The figure shows three views and two pictorial views of one solid part (mm, origin at its lowest corner). Answer the questions. Give positions to 0.01 mm unless a question says otherwise; leave off trailing zeros. Loops run counter-clockwise (first coordinate to the right, second up) from the corner with the lowest first, then second, coordinate; pieces in that order, holes last. Notation, with made-up numbers: M 56,-19 L 70,-19 A10 cw 70,-2 Z; hole C 73,12 d1. An arc over 180 degrees is marked long. Write item = value, one per line. Start each with the question number.
1. Section A-A on y = 1.05 is taken. Determine the outline of the cut face in (x, z).
2. Section B-B on z = 2 is taken. Determine the outline of the cut face in (x, y).
3. Consider L1, parallel to Z at x = 16, y = 0.7; L2, parallel to X at y = 0.2, z = 2.5; L3, parallel to Z at x = 38, y = 0.75. Determine where each line is inside the solid, lowest interval first. Write a range as [from, to].
4. Section D-D on x = 29 is taken. Determine the outline of the cut face in (y, z).
5. Section C-C on z = 5.25 is taken. Determine the outline of the cut face in (x, y).
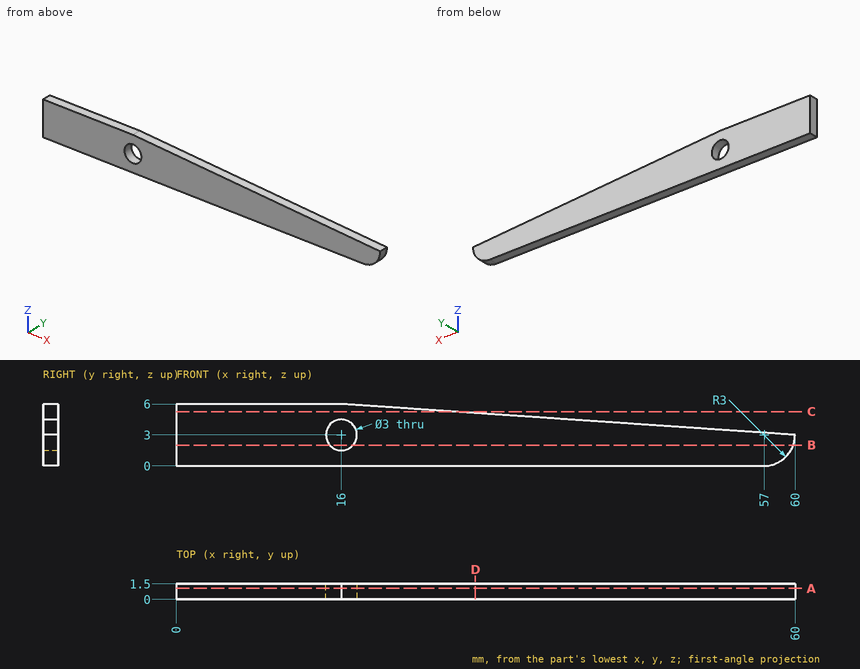
Verdict:
q1.outline = M 0,0 L 57,0 A3 ccw 60,3 L 16,6 L 0,6 Z; hole C 16,3 d3
q2.outline = M 0,0 L 14.88,0 L 14.88,1.5 L 0,1.5 Z; M 17.12,0 L 59.83,0 L 59.83,1.5 L 17.12,1.5 Z
q3.L1 = [0, 1.5], [4.5, 6]
q3.L2 = [0, 14.59], [17.41, 59.96]
q3.L3 = [0, 4.5]
q4.outline = M 0,0 L 1.5,0 L 1.5,5.11 L 0,5.11 Z
q5.outline = M 0,0 L 27,0 L 27,1.5 L 0,1.5 Z
